Geometry: final body of the model. Coordinates: model frame, mm. Round coordinates to 2 decimals unless told otherwise and drop trailing zeros. Loops run counter-clockwise (first coordinate to the right, second up) from the corner with the lowest first, then second, coordinate; pieces in that order, holes last. Notation, with made-up numbers: (53, 75.5) - (95, 75.5) arc R17 cw to (95, 103.5) - close; hole circle Ø3 at (4.25, -11.5). An arc over 180 degrees is marked (long way). Answer as CSV lines item,"result".
from build123d import *

# Parameters (mm, degrees)
SKETCH1_W                  = 500
SKETCH1_H                  = 1000
BOSS_EXTRUDE1_DEPTH        = 10
LO_BAT_XUONG_DAT_REACH     = 12
SKETCH2_R                  = 10
FILLET1_R                  = 10
CUT_EXTRUDE2_REACH         = 12
SKETCH3_R                  = 70.65
BAT_CHAN_DE_KHOP_NOI_REACH = 12
SKETCH4_R                  = 3
CUT_EXTRUDE3_REACH         = 12
SKETCH6_R                  = 3


with BuildPart() as part:
    # Sketch1 → Boss-Extrude1 (new body)
    with BuildSketch(Plane(origin=(0, 0, 0), x_dir=(1, 0, 0), z_dir=(0, 1, 0))):
        Rectangle(SKETCH1_W, SKETCH1_H)
    extrude(amount=BOSS_EXTRUDE1_DEPTH)

    # Sketch2 → lo bat xuong dat (cut, up to next)
    with BuildSketch(Plane(origin=(0, 10, 0), x_dir=(1, 0, 0), z_dir=(0, 1, 0)), mode=Mode.PRIVATE) as lo_bat_xuong_dat_sk1:
        with Locations((-225, 475)):
            Circle(SKETCH2_R)
    lo_bat_xuong_dat_tool1 = extrude(lo_bat_xuong_dat_sk1.sketch, amount=-LO_BAT_XUONG_DAT_REACH, mode=Mode.PRIVATE) & part.part
    add(lo_bat_xuong_dat_tool1.solids().sort_by_distance((-225, 10, -475))[0], mode=Mode.SUBTRACT)
    # Sketch2 → lo bat xuong dat (cut, up to next)
    with BuildSketch(Plane(origin=(0, 10, 0), x_dir=(1, 0, 0), z_dir=(0, 1, 0)), mode=Mode.PRIVATE) as lo_bat_xuong_dat_sk2:
        with Locations((225, 475)):
            Circle(SKETCH2_R)
    lo_bat_xuong_dat_tool2 = extrude(lo_bat_xuong_dat_sk2.sketch, amount=-LO_BAT_XUONG_DAT_REACH, mode=Mode.PRIVATE) & part.part
    add(lo_bat_xuong_dat_tool2.solids().sort_by_distance((225, 10, -475))[0], mode=Mode.SUBTRACT)
    # Sketch2 → lo bat xuong dat (cut, up to next)
    with BuildSketch(Plane(origin=(0, 10, 0), x_dir=(1, 0, 0), z_dir=(0, 1, 0)), mode=Mode.PRIVATE) as lo_bat_xuong_dat_sk3:
        with Locations((-225, -475)):
            Circle(SKETCH2_R)
    lo_bat_xuong_dat_tool3 = extrude(lo_bat_xuong_dat_sk3.sketch, amount=-LO_BAT_XUONG_DAT_REACH, mode=Mode.PRIVATE) & part.part
    add(lo_bat_xuong_dat_tool3.solids().sort_by_distance((-225, 10, 475))[0], mode=Mode.SUBTRACT)
    # Sketch2 → lo bat xuong dat (cut, up to next)
    with BuildSketch(Plane(origin=(0, 10, 0), x_dir=(1, 0, 0), z_dir=(0, 1, 0)), mode=Mode.PRIVATE) as lo_bat_xuong_dat_sk4:
        with Locations((225, -475)):
            Circle(SKETCH2_R)
    lo_bat_xuong_dat_tool4 = extrude(lo_bat_xuong_dat_sk4.sketch, amount=-LO_BAT_XUONG_DAT_REACH, mode=Mode.PRIVATE) & part.part
    add(lo_bat_xuong_dat_tool4.solids().sort_by_distance((225, 10, 475))[0], mode=Mode.SUBTRACT)

    # Fillet1
    fillet1_edges = [part.edges().sort_by_distance(p)[0] for p in [
        (250, 5, 500),
        (-250, 5, 500),
        (-250, 5, -500),
        (250, 5, -500),
    ]]
    fillet(fillet1_edges, radius=FILLET1_R)

    # Sketch3 → Cut-Extrude2 (cut, up to next)
    with BuildSketch(Plane(origin=(0, 10, 0), x_dir=(1, 0, 0), z_dir=(0, 1, 0)), mode=Mode.PRIVATE) as cut_extrude2_sk1:
        with Locations((0, 330)):
            Circle(SKETCH3_R)
    cut_extrude2_tool1 = extrude(cut_extrude2_sk1.sketch, amount=-CUT_EXTRUDE2_REACH, mode=Mode.PRIVATE) & part.part
    add(cut_extrude2_tool1.solids().sort_by_distance((0, 10, -330))[0], mode=Mode.SUBTRACT)

    # Sketch4 → bat chan de khop noi (cut, up to next)
    with BuildSketch(Plane(origin=(0, 10, 0), x_dir=(1, 0, 0), z_dir=(0, 1, 0)), mode=Mode.PRIVATE) as bat_chan_de_khop_noi_sk1:
        with Locations((-85, 120)):
            Circle(SKETCH4_R)
    bat_chan_de_khop_noi_tool1 = extrude(bat_chan_de_khop_noi_sk1.sketch, amount=-BAT_CHAN_DE_KHOP_NOI_REACH, mode=Mode.PRIVATE) & part.part
    add(bat_chan_de_khop_noi_tool1.solids().sort_by_distance((-85, 10, -120))[0], mode=Mode.SUBTRACT)
    # Sketch4 → bat chan de khop noi (cut, up to next)
    with BuildSketch(Plane(origin=(0, 10, 0), x_dir=(1, 0, 0), z_dir=(0, 1, 0)), mode=Mode.PRIVATE) as bat_chan_de_khop_noi_sk2:
        with Locations((85, 120)):
            Circle(SKETCH4_R)
    bat_chan_de_khop_noi_tool2 = extrude(bat_chan_de_khop_noi_sk2.sketch, amount=-BAT_CHAN_DE_KHOP_NOI_REACH, mode=Mode.PRIVATE) & part.part
    add(bat_chan_de_khop_noi_tool2.solids().sort_by_distance((85, 10, -120))[0], mode=Mode.SUBTRACT)
    # Sketch4 → bat chan de khop noi (cut, up to next)
    with BuildSketch(Plane(origin=(0, 10, 0), x_dir=(1, 0, 0), z_dir=(0, 1, 0)), mode=Mode.PRIVATE) as bat_chan_de_khop_noi_sk3:
        with Locations((85, -120)):
            Circle(SKETCH4_R)
    bat_chan_de_khop_noi_tool3 = extrude(bat_chan_de_khop_noi_sk3.sketch, amount=-BAT_CHAN_DE_KHOP_NOI_REACH, mode=Mode.PRIVATE) & part.part
    add(bat_chan_de_khop_noi_tool3.solids().sort_by_distance((85, 10, 120))[0], mode=Mode.SUBTRACT)
    # Sketch4 → bat chan de khop noi (cut, up to next)
    with BuildSketch(Plane(origin=(0, 10, 0), x_dir=(1, 0, 0), z_dir=(0, 1, 0)), mode=Mode.PRIVATE) as bat_chan_de_khop_noi_sk4:
        with Locations((-85, -120)):
            Circle(SKETCH4_R)
    bat_chan_de_khop_noi_tool4 = extrude(bat_chan_de_khop_noi_sk4.sketch, amount=-BAT_CHAN_DE_KHOP_NOI_REACH, mode=Mode.PRIVATE) & part.part
    add(bat_chan_de_khop_noi_tool4.solids().sort_by_distance((-85, 10, 120))[0], mode=Mode.SUBTRACT)

    # Sketch6 → Cut-Extrude3 (cut, up to next)
    with BuildSketch(Plane(origin=(0, 10, 0), x_dir=(1, 0, 0), z_dir=(0, 1, 0)), mode=Mode.PRIVATE) as cut_extrude3_sk1:
        with Locations((238, -375)):
            Circle(SKETCH6_R)
    cut_extrude3_tool1 = extrude(cut_extrude3_sk1.sketch, amount=-CUT_EXTRUDE3_REACH, mode=Mode.PRIVATE) & part.part
    add(cut_extrude3_tool1.solids().sort_by_distance((238, 10, 375))[0], mode=Mode.SUBTRACT)
    # Sketch6 → Cut-Extrude3 (cut, up to next)
    with BuildSketch(Plane(origin=(0, 10, 0), x_dir=(1, 0, 0), z_dir=(0, 1, 0)), mode=Mode.PRIVATE) as cut_extrude3_sk2:
        with Locations((102, -375)):
            Circle(SKETCH6_R)
    cut_extrude3_tool2 = extrude(cut_extrude3_sk2.sketch, amount=-CUT_EXTRUDE3_REACH, mode=Mode.PRIVATE) & part.part
    add(cut_extrude3_tool2.solids().sort_by_distance((102, 10, 375))[0], mode=Mode.SUBTRACT)
    # Sketch6 → Cut-Extrude3 (cut, up to next)
    with BuildSketch(Plane(origin=(0, 10, 0), x_dir=(1, 0, 0), z_dir=(0, 1, 0)), mode=Mode.PRIVATE) as cut_extrude3_sk3:
        with Locations((-102, -375)):
            Circle(SKETCH6_R)
    cut_extrude3_tool3 = extrude(cut_extrude3_sk3.sketch, amount=-CUT_EXTRUDE3_REACH, mode=Mode.PRIVATE) & part.part
    add(cut_extrude3_tool3.solids().sort_by_distance((-102, 10, 375))[0], mode=Mode.SUBTRACT)
    # Sketch6 → Cut-Extrude3 (cut, up to next)
    with BuildSketch(Plane(origin=(0, 10, 0), x_dir=(1, 0, 0), z_dir=(0, 1, 0)), mode=Mode.PRIVATE) as cut_extrude3_sk4:
        with Locations((-238, -375)):
            Circle(SKETCH6_R)
    cut_extrude3_tool4 = extrude(cut_extrude3_sk4.sketch, amount=-CUT_EXTRUDE3_REACH, mode=Mode.PRIVATE) & part.part
    add(cut_extrude3_tool4.solids().sort_by_distance((-238, 10, 375))[0], mode=Mode.SUBTRACT)
    # Sketch6 → Cut-Extrude3 (cut, up to next)
    with BuildSketch(Plane(origin=(0, 10, 0), x_dir=(1, 0, 0), z_dir=(0, 1, 0)), mode=Mode.PRIVATE) as cut_extrude3_sk5:
        with Locations((-238, 375)):
            Circle(SKETCH6_R)
    cut_extrude3_tool5 = extrude(cut_extrude3_sk5.sketch, amount=-CUT_EXTRUDE3_REACH, mode=Mode.PRIVATE) & part.part
    add(cut_extrude3_tool5.solids().sort_by_distance((-238, 10, -375))[0], mode=Mode.SUBTRACT)
    # Sketch6 → Cut-Extrude3 (cut, up to next)
    with BuildSketch(Plane(origin=(0, 10, 0), x_dir=(1, 0, 0), z_dir=(0, 1, 0)), mode=Mode.PRIVATE) as cut_extrude3_sk6:
        with Locations((-102, 375)):
            Circle(SKETCH6_R)
    cut_extrude3_tool6 = extrude(cut_extrude3_sk6.sketch, amount=-CUT_EXTRUDE3_REACH, mode=Mode.PRIVATE) & part.part
    add(cut_extrude3_tool6.solids().sort_by_distance((-102, 10, -375))[0], mode=Mode.SUBTRACT)
    # Sketch6 → Cut-Extrude3 (cut, up to next)
    with BuildSketch(Plane(origin=(0, 10, 0), x_dir=(1, 0, 0), z_dir=(0, 1, 0)), mode=Mode.PRIVATE) as cut_extrude3_sk7:
        with Locations((102, 375)):
            Circle(SKETCH6_R)
    cut_extrude3_tool7 = extrude(cut_extrude3_sk7.sketch, amount=-CUT_EXTRUDE3_REACH, mode=Mode.PRIVATE) & part.part
    add(cut_extrude3_tool7.solids().sort_by_distance((102, 10, -375))[0], mode=Mode.SUBTRACT)
    # Sketch6 → Cut-Extrude3 (cut, up to next)
    with BuildSketch(Plane(origin=(0, 10, 0), x_dir=(1, 0, 0), z_dir=(0, 1, 0)), mode=Mode.PRIVATE) as cut_extrude3_sk8:
        with Locations((238, 375)):
            Circle(SKETCH6_R)
    cut_extrude3_tool8 = extrude(cut_extrude3_sk8.sketch, amount=-CUT_EXTRUDE3_REACH, mode=Mode.PRIVATE) & part.part
    add(cut_extrude3_tool8.solids().sort_by_distance((238, 10, -375))[0], mode=Mode.SUBTRACT)
    # Sketch6 → Cut-Extrude3 (cut, up to next)
    with BuildSketch(Plane(origin=(0, 10, 0), x_dir=(1, 0, 0), z_dir=(0, 1, 0)), mode=Mode.PRIVATE) as cut_extrude3_sk9:
        with Locations((68, -375)):
            Circle(SKETCH6_R)
    cut_extrude3_tool9 = extrude(cut_extrude3_sk9.sketch, amount=-CUT_EXTRUDE3_REACH, mode=Mode.PRIVATE) & part.part
    add(cut_extrude3_tool9.solids().sort_by_distance((68, 10, 375))[0], mode=Mode.SUBTRACT)
    # Sketch6 → Cut-Extrude3 (cut, up to next)
    with BuildSketch(Plane(origin=(0, 10, 0), x_dir=(1, 0, 0), z_dir=(0, 1, 0)), mode=Mode.PRIVATE) as cut_extrude3_sk10:
        with Locations((-68, -375)):
            Circle(SKETCH6_R)
    cut_extrude3_tool10 = extrude(cut_extrude3_sk10.sketch, amount=-CUT_EXTRUDE3_REACH, mode=Mode.PRIVATE) & part.part
    add(cut_extrude3_tool10.solids().sort_by_distance((-68, 10, 375))[0], mode=Mode.SUBTRACT)


solid = part.part
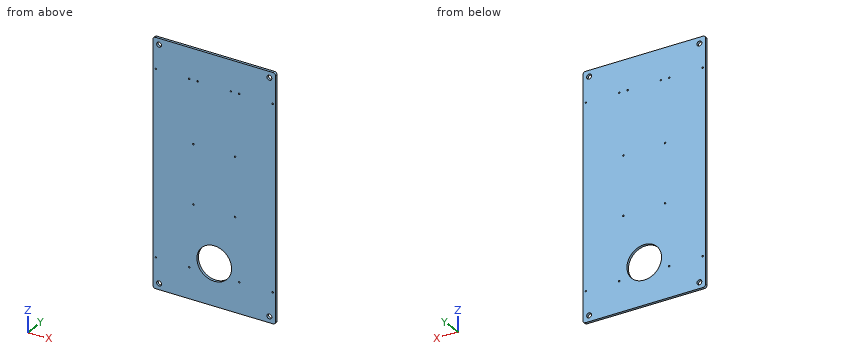
(1) Pin query (flat end, axial travel): P1, Ø5, axis at x = -68, z = 375, coming from the +Y side. Return the tip coordinate at first contact, or that it passes through.
Findings below:
P1,"through"
(2) Section A-A (z = -330). Output: boundary loops of the cut face in (x, y), and give its area (3 significant figures).
Findings below:
outline,"(-250, 0) - (-70.65, 0) - (-70.65, 10) - (-250, 10) - close; (70.65, 0) - (250, 0) - (250, 10) - (70.65, 10) - close"
area,"3,590 mm2"
(3) Section B-B (y = 7). Give the number of separate pieces and of enclosed holes in the cut face, and give its area (3 significant figures).
Findings below:
separate pieces,"1"
enclosed holes,"19"
area,"483,000 mm2"
(4) Material intervals for line 1 along X through (y, z) = (2.5, 120); line 2 along Z through (x, y) = (85, 4.25); line 3 along X through (y, z) = (6.25, -475), sorted ascending.
Findings below:
line 1,"-250 to -88, -82 to 82, 88 to 250"
line 2,"-500 to -123, -117 to 117, 123 to 500"
line 3,"-250 to -235, -215 to 215, 235 to 250"
